Read the model definition and answer for the solid it produces. Units are mm, in the model's axes. Coordinates: 2 decimals unless noted, no trailing zeros. Loops run counter-clockwise (first coordinate to the right, second up) from the corner with the lowest first, then second, coordinate; pieces in that order, holes last.
Q1. Section B-B (x = 0.4) is taken. Count the separate pieces of the cut face and the enclosed holes in it, then the cut area to 3 significant figures.
Q2. Straight lines are drawn through the part: line 1 (Y direction, x = 0.15, z = 28.5) (3 decimals); line 2 (Y direction, x = 0.25, z = -27) (3 decimals); line 3 (Z direction, x = 1.9, y = 29.5). For each, find the intervals that lie inside material, in ascending order.
Q3. The mould has two halves that part along Y. Classify faces 1 (the face through (1.03, 3.62, -53.33)), 2 (the face through (1, 18.89, 147.42)), 3 (the face through (1.002, 17.672, 119.067)), 4 (the face through (1.03, 31.303, -53.331)): pulls with the +Y half, pulls with the -Y half, needs draft (parallel to the pull), parting line crosses it, or undercut.
Q4. Section A-A (z = -7.5) is taken. Give the vertices of the cut face in (x, y) (3 decimals), then the cut area to 3 significant figures.
Q5. Flat-ended cylindrical pins translate along their axes: P1, Ø12.5, axis at y = 17.46, z = 123.82, coming from the -X side; P2, Ø5.5, axis at y = 17.46, z = 47.62, coming from the -X side. Find the tip coordinate at first contact, or state that the pin passes through.
Q6. Section D-D (y = 30) is taken. Give the vertices of the cut face in (x, z).
from build123d import *

# Parameters (mm, degrees)
SKETCH1_W           = 2.032
SKETCH1_H           = 34.925
BOSS_EXTRUDE1_DEPTH = 152.4
CUT_EXTRUDE1_REACH  = 158.364
SKETCH2_R           = 4.7625
LPATTERN1_COUNT     = 16
LPATTERN1_PITCH     = 19.05
SKETCH4_W           = 2.032
SKETCH4_H           = 34.925
CUT_EXTRUDE2_DEPTH  = 213.450199221
FILLET1_R           = 12.7


with BuildPart() as part:
    # Sketch1 → Boss-Extrude1 (new, symmetric)
    with BuildSketch(Plane.XY):
        with Locations((1.016, 17.4625)):
            Rectangle(SKETCH1_W, SKETCH1_H)
    extrude(amount=BOSS_EXTRUDE1_DEPTH, both=True)

    # Sketch2 → Cut-Extrude1 (cut, up to next)
    with BuildSketch(Plane.ZY, mode=Mode.PRIVATE) as cut_extrude1_sk1:
        with Locations((142.875, 17.4625)):
            Circle(SKETCH2_R)
    cut_extrude1_tool1 = extrude(cut_extrude1_sk1.sketch, amount=-CUT_EXTRUDE1_REACH, mode=Mode.PRIVATE) & part.part
    cut_extrude1 = cut_extrude1_tool1.solids().sort_by_distance((0, 17.4625, 142.875))[0]
    add(cut_extrude1, mode=Mode.SUBTRACT)

    # LPattern1: Cut-Extrude1 ×16
    with Locations(*[(0, 0, -i * LPATTERN1_PITCH) for i in range(1, LPATTERN1_COUNT)]):
        add(cut_extrude1, mode=Mode.SUBTRACT)

    # Sketch4 → Cut-Extrude2 (cut, through all)
    with BuildSketch(Plane.XY.offset(-57.15)):
        with Locations((1.016, 17.4625)):
            Rectangle(SKETCH4_W, SKETCH4_H)
    extrude(amount=-CUT_EXTRUDE2_DEPTH, mode=Mode.SUBTRACT)

    # Fillet1
    fillet1_edges = [part.edges().sort_by_distance(p)[0] for p in [
        (1.016, 34.925, 152.4),
        (1.016, 0, -57.15),
        (1.016, 34.925, -57.15),
        (1.016, 0, 152.4),
    ]]
    fillet(fillet1_edges, radius=FILLET1_R)


solid = part.part
Numbers:
1. separate pieces: 1
1. enclosed holes: 11
1. area: 6,400 mm2
2. line 1: y = 0 to 12.701, 22.224 to 34.925
2. line 2: y = 0 to 12.968, 21.957 to 34.925
2. line 3: z = -54.86 to 150.11
3. face 1: pulls with the -Y half
3. face 2: undercut
3. face 3: undercut
3. face 4: pulls with the +Y half
4. outline: (0, 0) - (2.032, 0) - (2.032, 13.152) - (0, 13.152) - close; (0, 21.773) - (2.032, 21.773) - (2.032, 34.925) - (0, 34.925) - close
4. area: 53.4 mm2
5. P1: stops at x = 0
5. P2: passes through
6. outline: (0, -54.49) - (2.03, -54.49) - (2.03, 149.74) - (0, 149.74) - close
